Design review of the part built by this model. Coordinates are the model's own, in mm. Face numbers are marked on the shaded views. A direction names the side the tool comes from. Give positions to 0.01 mm unless a question says otherwise; leave off trailing zeros. Loops run counter-clockwise (first coordinate to the right, second up) from the corner with the lowest first, then second, coordinate; pieces in that order, holes last. Notation, with made-up numbers: (58, 18.5) - (79, 18.5) arc R21 cw to (79, 47.5) - close; hole circle Ø6 at (-33.75, 85). An arc over 180 degrees is marked (long way). Put each result on its own line as item: value. Start each with the question number.
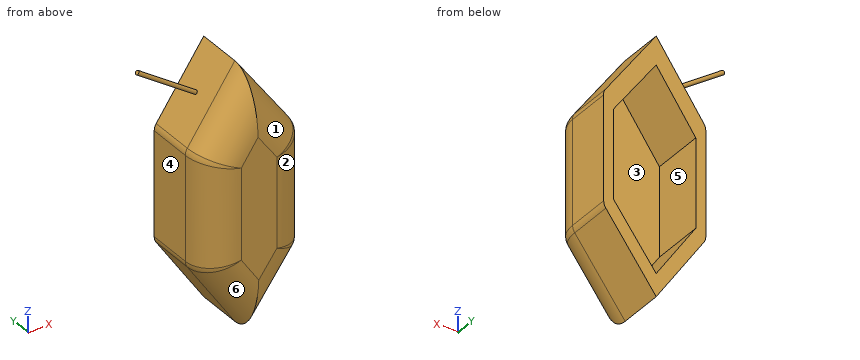
```python
from build123d import *

# Parameters (mm, degrees)
BOSS_EXTRUDE1_DEPTH = 71
CUT_EXTRUDE1_DEPTH  = 48
FILLET1_R           = 30
FILLET2_R           = 10
SKETCH3_R           = 1.773463316
BOSS_EXTRUDE2_DEPTH = 64


with BuildPart() as part:
    # Sketch1 → Boss-Extrude1 (new body)
    with BuildSketch(Plane(origin=(0, 0, 0), x_dir=(1, 0, 0), z_dir=(0, 1, 0))):
        Polygon((-53.484564952, 104.184508732), (-98.158322107, 37.819944229), (-98.158322107, -62.180055771), (-53.484564952, -126.659696939), (-5.888781519, -60.295132437), (-6.131233796, 39.704573647), align=None)
    extrude(amount=BOSS_EXTRUDE1_DEPTH)

    # Sketch2 → Cut-Extrude1 (cut)
    with BuildSketch(Plane(origin=(0, 71, 0), x_dir=(1, 0, 0), z_dir=(0, 1, 0))):
        Polygon((-53.419316383, 83.690098923), (-89.158322107, 30.598447321), (-89.158322107, -49.401552679), (-53.419316383, -100.985265614), (-14.918881702, -47.891189489), (-15.112843524, 32.108575378), align=None)
    extrude(amount=-CUT_EXTRUDE1_DEPTH, mode=Mode.SUBTRACT)

    # Fillet1
    fillet1_edges = [part.edges().sort_by_distance(p)[0] for p in [
        (-6.010007658, 0, 10.295279395),
        (-29.686673235, 0, 93.477414688),
        (-75.821443529, 0, 94.419876355),
        (-98.158322107, 0, 12.180055771),
        (-75.821443529, 0, -71.002226481),
        (-29.807899374, 0, -71.94454119),
    ]]
    fillet(fillet1_edges, radius=FILLET1_R)

    # Fillet2
    fillet2_edges = [part.edges().sort_by_distance(p)[0] for p in [
        (-6.131233796, 50.5, -39.704573647),
        (-5.888781519, 50.5, 60.295132437),
        (-98.158322107, 50.5, 62.180055771),
        (-98.158322107, 50.5, -37.819944229),
        (-15.180720611, 8.520303105, -36.726448686),
        (-14.946943145, 8.525742818, 57.394836212),
        (-89.134201731, 8.55209861, -35.065579718),
        (-89.123112182, 8.541258724, 59.355901315),
    ]]
    fillet(fillet2_edges, radius=FILLET2_R)

    # Sketch3 → Boss-Extrude2 (add)
    with BuildSketch(Plane(origin=(-95.430334367, 0, 66.117483062), x_dir=(0.569502992, 0, 0.821989259), z_dir=(-0.821989259, 0, 0.569502992))):
        with Locations((35.994445749, 50.5)):
            Circle(SKETCH3_R)
    extrude(amount=BOSS_EXTRUDE2_DEPTH)


solid = part.part
```
Item 1: Mouldability with a two-part tool opening along Z and no side actions: class the marked faces 4, 5 and 6 as pulls with the +Z half, pulls with the -Z half, needs draft (parallel to the pull), parting line crosses it, or undercut.
Item 2: Machinability: for the marked faces 1, 2 and 3, which of the approach directions +Z, -Z, +X, -X, +Y, -Y give a long, thin tool a straight path to every point of the face, cutting with its end or side? Answer none if there is none.
Item 3: For L1, parallel to X at y = 48.5, z = -29; L2, parallel to Z at x = -21, y = 35; L3, parallel to Z at x = -77, y = 47, list the stretches that pass through material, from the lowest coordinate up. Write a range as from..to.
Item 4: For P1, Ø5, axis at x = -32.5, z = -10, coming from the +Y side; P2, Ø1, axis at x = -94, y = 23.5, coming from the +Z side; P3, Ø4, axis at x = -30, y = 48, coming from the +Z side, all flat-tipped, find the tip position at first contact; note any pin that passes through.
Item 5: Consider section A-A (y = 42). State the section outline as (x, z) points, plus the area to 3 significant figures.
Geometry says:
1. face 4: needs draft
1. face 5: undercut
1. face 6: pulls with the -Z half
2. face 1: +Z, +X, -Y
2. face 2: -Z, +X, -Y
2. face 3: +Y
3. L1: x = -98.16..-89.16, -15.11..-6.11
3. L2: z = -59.95..-40.04, 56.28..81.37
3. L3: z = -69.25..-48.66, 66.95..92.72
4. P1: stops at y = 23
4. P2: stops at z = 67.68
4. P3: stops at z = 96.7
5. outline: (-98.16, -34.77) arc R10 ccw to (-96.45, -40.35) - (-53.48, -104.18) - (-8.06, -42.34) arc R10 ccw to (-6.12, -36.44) - (-5.9, 57.07) arc R10 ccw to (-7.77, 62.92) - (-53.48, 126.66) - (-96.38, 64.75) arc R10 ccw to (-98.16, 59.05) - close; hole (-89.16, -30.6) - (-53.42, -83.69) - (-15.11, -32.11) - (-14.92, 47.89) - (-53.42, 100.99) - (-89.16, 49.4) - close
5. area: 5,430 mm2
